```python
from build123d import *
from OCP.BRepFilletAPI import BRepFilletAPI_MakeChamfer

# Parameters (mm, degrees)
SKETCH1_W           = 36.5
SKETCH1_H           = 19.2
BOSS_EXTRUDE1_DEPTH = 5
SKETCH2_R           = 1
SKETCH2_W           = 23
SKETCH2_H           = 15.7
CUT_EXTRUDE3_DEPTH  = 67.428509309
SKETCH4_W           = 60
SKETCH4_H           = 15
BOSS_EXTRUDE2_DEPTH = 0.5
BOSS_EXTRUDE3_DEPTH = 3.5
CHAMFER1_SIZE       = 2
CHAMFER2_SIZE       = 1
CHAMFER3_SIZE       = 4
CHAMFER3_SIZE2      = 2.309401077
FILLET1_R           = 2
CUT_EXTRUDE4_DEPTH  = 1
FILLET2_R           = 1
CUT_EXTRUDE5_DEPTH  = 10
CHAMFER4_SIZE       = 1


with BuildPart() as part:
    # Sketch1 → Boss-Extrude1 (new body)
    with BuildSketch(Plane.XY):
        with Locations((-1.102631579, 53.75)):
            Rectangle(SKETCH1_W, SKETCH1_H)
    extrude(amount=BOSS_EXTRUDE1_DEPTH)

    # Sketch2 → Cut-Extrude3 (cut, through all)
    with BuildSketch(Plane.XY.offset(5)):
        with Locations((-15.252631579, 53.75)):
            Circle(SKETCH2_R)
        with Locations((12.547368421, 53.75)):
            Circle(SKETCH2_R)
        with Locations((-1.352631579, 52)):
            Rectangle(SKETCH2_W, SKETCH2_H)
    extrude(amount=-CUT_EXTRUDE3_DEPTH, mode=Mode.SUBTRACT)

    # Sketch4 → Boss-Extrude2 (add)
    with BuildSketch(Plane(origin=(0, 63.35, 0), x_dir=(1, 0, 0), z_dir=(0, 1, 0))):
        with Locations((-12.852631579, -7.5)):
            Rectangle(SKETCH4_W, SKETCH4_H)
    extrude(amount=BOSS_EXTRUDE2_DEPTH)

    # Sketch7 → Boss-Extrude3 (add)
    with BuildSketch(Plane.XZ.offset(-63.35)):
        Polygon((-19.352631579, 0), (-42.852631579, 0), (-42.852631579, 15), (-19.052631579, 15), (17.147368421, 15), (17.147368421, 5), (-19.352631579, 5), align=None)
    extrude(amount=BOSS_EXTRUDE3_DEPTH)

    # Chamfer1
    chamfer1_edges = [part.edges().sort_by_distance(p)[0] for p in [
        (-12.852631579, 59.85, 15),
    ]]
    chamfer(chamfer1_edges, length=CHAMFER1_SIZE)

    # Chamfer2
    chamfer2_edges = [part.edges().sort_by_distance(p)[0] for p in [
        (-12.852631579, 44.15, 2.5),
        (10.147368421, 44.15, 2.5),
        (17.147368421, 63.85, 7.5),
        (-12.852631579, 63.85, 0),
        (-12.852631579, 63.85, 15),
        (-19.352631579, 59.85, 2.5),
        (-19.352631579, 44.15, 2.5),
    ]]
    chamfer(chamfer2_edges, length=CHAMFER2_SIZE)

    # Chamfer3: one chamfer whose edges measure the first distance from different faces: ONE call of the kernel's chamfer builder (chamfer() names one face for all edges)
    chamfer3_edges_1 = [part.edges().sort_by_distance(p)[0] for p in [
        (-42.852631579, 61.35, 0),
    ]]
    chamfer3_side_1 = [part.faces().sort_by_distance(p)[0] for p in [
        (-18.724165987, 52, 0),
    ]]
    chamfer3_edges_2 = [part.edges().sort_by_distance(p)[0] for p in [
        (-42.852631579, 62.35, 15),
    ]]
    chamfer3_side_2 = [part.faces().sort_by_distance(p)[0] for p in [
        (-42.852631579, 61.86754386, 7.260233918),
    ]]
    chamfer3 = BRepFilletAPI_MakeChamfer(part.part.solid().wrapped)
    for e in chamfer3_edges_1:
        chamfer3.Add(CHAMFER3_SIZE, CHAMFER3_SIZE2, e.wrapped, chamfer3_side_1[0].wrapped)  # the first distance lies on this face
    for e in chamfer3_edges_2:
        chamfer3.Add(CHAMFER3_SIZE, CHAMFER3_SIZE2, e.wrapped, chamfer3_side_2[0].wrapped)  # the first distance lies on this face
    add(Compound.cast(chamfer3.Shape()), mode=Mode.REPLACE)

    # Fillet1
    fillet1_edges = [part.edges().sort_by_distance(p)[0] for p in [
        (-42.852631579, 61.85, 11),
        (-42.852631579, 61.85, 2.309401077),
    ]]
    fillet(fillet1_edges, radius=FILLET1_R)

    # Sketch8 → Cut-Extrude4 (cut)
    with BuildSketch(Plane(origin=(0, 63.85, 0), x_dir=(1, 0, 0), z_dir=(0, 1, 0))):
        Polygon((-0.652631579, -2), (-2.817695088, -5.75), (1.512431931, -5.75), align=None)
    extrude(amount=-CUT_EXTRUDE4_DEPTH, mode=Mode.SUBTRACT)

    # Fillet2
    fillet2_edges = [part.edges().sort_by_distance(p)[0] for p in [
        (-41.218656983, 63.85, 1.366025404),
        (-42.584682387, 63.85, 2.464101615),
        (-41.852631579, 63.85, 12.732050808),
        (-42.784483232, 63.85, 10.981739705),
        (-40.352631579, 59.85, 0.866025404),
        (-42.584682387, 59.85, 2.464101615),
        (-42.141306714, 59.85, 12.232050808),
        (-42.784483232, 59.85, 10.981739705),
        (-42.852631579, 63.85, 6.964101615),
        (-42.852631579, 59.85, 6.964101615),
    ]]
    fillet(fillet2_edges, radius=FILLET2_R - 0.0001)  # a hair under: the kernel refuses the full size

    # Sketch9 → Cut-Extrude5 (cut)
    with BuildSketch(Plane(origin=(0, 63.85, 0), x_dir=(1, 0, 0), z_dir=(0, 1, 0))):
        Polygon((17.147368421, -5), (10.647368421, -5), (10.647368421, -10), (-23.452631579, -10), (-23.452631579, -15), (9.647368421, -15), (17.147368421, -15), align=None)
    extrude(amount=-CUT_EXTRUDE5_DEPTH, mode=Mode.SUBTRACT)

    # Chamfer4
    chamfer4_edges = [part.edges().sort_by_distance(p)[0] for p in [
        (10.647368421, 61.85, 5),
        (-23.452631579, 61.85, 10),
        (10.647368421, 61.85, 10),
        (-23.452631579, 62.35, 15),
    ]]
    chamfer(chamfer4_edges, length=CHAMFER4_SIZE)


solid = part.part
```
The model under review builds one solid part; all positions refer to its coordinate system, in mm. A direction names the side the tool comes from. Coordinates: 2 decimals unless noted, no trailing zeros. Write each loop counter-clockwise with the first axis right and the second up, starting at its lowest first coordinate (ties: lowest second). Pieces come first, ordered by that corner, then holes. Notation, with made-up numbers: (44, -34) - (54, -34) arc R16 cw to (54, -26) - close; hole circle Ø1 at (42, 8.5). An arc over 180 degrees is marked (long way). Answer in a Markdown table with one row per item. Add a question column.
Q1. Consider section C-C on x = -35. Give the boundary of the cut face in (y, z).
Q2. Draft analysis for pull direction X (two halves, no side actions). For faces 1 (the face through (-23.453, 62, 12)), 2 (the face through (-11.57, 63.36, 0.51)), 3 (the face through (-0.7, 63.4, 5.75)), state which applies: +X half, -X half, draft (parallel to the pull), parting line (faces both ways), or undercut.
Q3. For faces 4 (the face through (10.7, 44.6, 2.5)), 5 (the face through (14, 54, 5)), 6 (the face through (-6, 62, 10)), 7 (the face through (-1, 62.85, 4)), list the 3-axis set-ups (+Z, -Z, +X, -X, +Y, -Y) from which the entire face can be reached by the end or side of a thin tool; tool diameter is ignored.
Q4. To check wall thickness, follow line 1 along X through (y, z) = (54, 4.75); line 2 along X through (y, z) = (51.75, 4); line 3 along X through (y, z) = (53.25, 2.5). State the ranges of each line that lie inside material, in increasing order. Write a range as from..to.
Q5. Clearance check with flat-ended pins moving along their axes: pin 1 (3 mm diameter, centred on x = -9.5, y = 61, fed in from +Z); pin 2 (1.1 mm diameter, centred on x = -1, y = 63.5, fed in from -Z); pin 3 (1.5 mm diameter, centred on x = -24.5, z = 5, fed in from -Y). State where each tip first meets the part, or that it passes through.
Q6. Consider section A-A on y = 53.75. Give the boundary of the cut face in (x, z).
Q7. Consider section D-D on z = 8. Give the boundary of the cut face in (x, y), then the cut area to 3 significant figures.
Q8. Consider section B-B on y = 46. Give the boundary of the cut face in (x, z), then the cut area to 3 significant figures.
Answers below:
| question | item | result |
|---|---|---|
| 1 | outline | (59.85, 0) - (62.85, 0) - (63.85, 1) - (63.85, 14) - (62.85, 15) - (61.85, 15) - (59.85, 13) - close |
| 2 | face 1 | +X half |
| 2 | face 2 | draft |
| 2 | face 3 | undercut |
| 3 | face 4 | +Z, -Z, -Y |
| 3 | face 5 | +Z, +X, -Y |
| 3 | face 6 | +Z, +X, +Y, -Y |
| 3 | face 7 | +Y |
| 4 | line 1 | -19.35..-16.22, -14.28..-12.85, 10.15..11.58, 13.52..17.15 |
| 4 | line 2 | -19.35..-12.85, 10.15..17.15 |
| 4 | line 3 | -19.35..-16.12, -14.39..-12.85, 10.15..11.68, 13.41..17.15 |
| 5 | pin 1 | z = 10 |
| 5 | pin 2 | z = 0.1 |
| 5 | pin 3 | y = 59.85 |
| 6 | outline | (-19.35, 0) - (-16.25, 0) - (-16.25, 5) - (-19.35, 5) - close; (-14.25, 0) - (-12.85, 0) - (-12.85, 5) - (-14.25, 5) - close; (10.15, 0) - (11.55, 0) - (11.55, 5) - (10.15, 5) - close; (13.55, 0) - (17.15, 0) - (17.15, 5) - (13.55, 5) - close |
| 7 | outline | (-42.85, 60.85) arc R1 ccw to (-41.85, 59.85) - (10.65, 59.85) - (10.65, 63.85) - (-41.85, 63.85) arc R1 ccw to (-42.85, 62.85) - close |
| 7 | area | 214 mm² |
| 8 | outline | (-19.35, 0) - (-12.85, 0) - (-12.85, 5) - (-19.35, 5) - close; (10.15, 0) - (17.15, 0) - (17.15, 5) - (10.15, 5) - close |
| 8 | area | 67.5 mm² |
